Read the model definition and answer for the solid it produces. Units are mm, in the model's axes. Face numbers are marked on the shaded views. A direction names the side the tool comes from. Give positions to 0.01 mm unless a question says otherwise; leave off trailing zeros. Order: outer loops, then holes, each group sorted by start corner. A loop starts at its lowest first (then second) coordinate and runs counter-clockwise, first axis right, second up. Notation, with made-up numbers: (79, 0) - (96, 0) arc R16 cw to (96, 15) - close; hole circle Ø1 at (-25, 17). An arc over 180 degrees is marked (long way). Return JSON: item names as keys, results as strings.
Autodesk Inventor part; units mm, degrees
ref_plane "YZ Plane" through (0, 0, 0) normal (1, 0, 0) x (0, 1, 0)
ref_plane "XZ Plane" through (0, 0, 0) normal (0, 1, 0) x (-1, 0, 0)
ref_plane "XY Plane" through (0, 0, 0) normal (0, 0, 1) x (1, 0, 0)
sketch "草圖1" plane through (0, 0, 0) normal (0, 1, 0) x (-1, 0, 0)
  line L0 (0, 0) -> (44.45, 0)
  line L1 (44.45, 0) -> (44.45, -44.45)
  line L2 (44.45, -44.45) -> (0, -44.45)
  line L3 (0, -44.45) -> (0, 0)
  line L4 (3.725, -3.725) -> (40.725, -3.725)
  line L5 (40.725, -3.725) -> (40.725, -40.725)
  line L6 (40.725, -40.725) -> (3.725, -40.725)
  line L7 (3.725, -40.725) -> (3.725, -3.725)
  circle A0 centre (40.725, -3.725) radius 1.6
  circle A1 centre (40.725, -40.725) radius 1.6
  circle A2 centre (3.725, -3.725) radius 1.6
  circle A3 centre (3.725, -40.725) radius 1.6
  line L8 (11, -33.725) -> (0, -33.725)
  line L9 (0, -33.725) -> (0, -10.725)
  line L10 (0, -10.725) -> (11, -10.725)
  line L11 (11, -10.725) -> (11, -33.725)
  point P0 (0, -33.725)
  dimension "d0" = 44.45
  dimension "d1" = 44.45
  dimension "d2" = 37
  dimension "d3" = 37
  dimension "d4" = 3.725
  dimension "d5" = 3.725
  dimension "d6" = 3.2
  dimension "d7" = 3.2
  dimension "d8" = 3.2
  dimension "d9" = 3.2
  dimension "d14" = 23
  dimension "d15" = 11
  dimension "d16" = 10.725
extrude "擠出1" add sketch "草圖1" along normal blind 27 contours L10 L7 L8 L3 | L10 L11 L8 L7
extrude "擠出2" cut sketch "草圖1" along normal blind 27 contours A2 L4 L7 | L7 L4 A2 | A3 L6 L7 | L7 L6 A3 | A0 L5 L4 | L4 L5 A0 | A1 L5 L6 | L6 L5 A1
extrude "擠出3" add sketch "草圖1" along normal blind 1.6 contours L0 L1 L2 L3 L8 L7 A3 L6 A1 L5 A0 L4 A2 L10 | L7 A2 L4 A0 L5 A1 L6 A3 L8 L11 L10
properties part number "l298n"
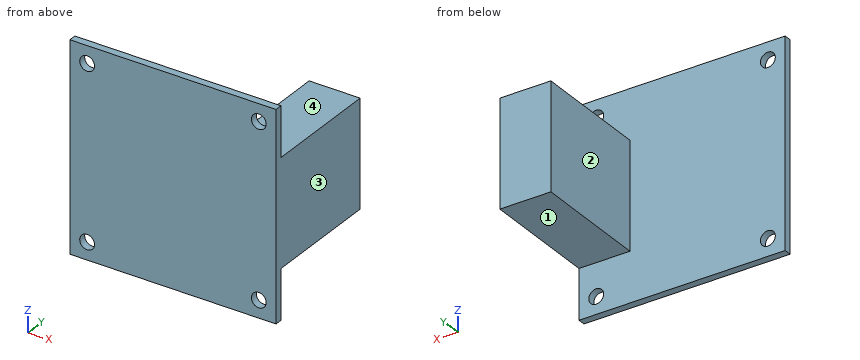
Q1. A cutting plane is placed at D-D (y = 10.75). Write down the section's boundary in (x, z) (3 decimals).
Values:
{"outline": "(-11, -33.725) - (0, -33.725) - (0, -10.725) - (-11, -10.725) - close"}
Q2. For the marked faces 1, 2, 3 and 4, determine the directions among +Z, -Z, +X, -X, +Y, -Y from which every point of the face is accessible in a straight line to the end or side of a thin tool.
Values:
{"face 1": "-Z, +X, -X, +Y", "face 2": "+Z, -Z, -X, +Y", "face 3": "+Z, -Z, +X, +Y, -Y", "face 4": "+Z, +X, -X, +Y"}
Q3. A cutting plane is placed at A-A (x = -4). Write down the section's boundary in (y, z) (3 decimals).
Values:
{"outline": "(0, -44.45) - (1.6, -44.45) - (1.6, -42.301) - (0, -42.301) - close; (0, -39.149) - (1.6, -39.149) - (1.6, -33.725) - (27, -33.725) - (27, -10.725) - (1.6, -10.725) - (1.6, -5.301) - (0, -5.301) - close; (0, -2.149) - (1.6, -2.149) - (1.6, 0) - (0, 0) - close"}
Q4. A cutting plane is placed at C-C (x = -38.5). Write down the section's boundary in (y, z), and give its area (3 significant figures).
Values:
{"outline": "(0, -44.45) - (1.6, -44.45) - (1.6, 0) - (0, 0) - close", "area": "71.1 mm²"}
Q5. Consider L1, parallel to Z at x = -40.5, y = 1.5; L2, parallel to Y at x = -33.5, z = -27; L3, parallel to Z at x = -5.5, y = 26 (3 decimals). Determine where each line is inside the solid, lowest interval first.
Values:
{"L1": "z = -44.45 to -42.31, -39.14 to -5.31, -2.14 to 0", "L2": "y = 0 to 1.6", "L3": "z = -33.725 to -10.725"}
Q6. Given pin 1 (1 mm diameter, centred on x = -29.5, z = -21.5, fed in from +Y); pin 2 (1.5 mm diameter, centred on x = -11.5, y = 9, fed in from -Z) (3 decimals); pin 3 (2 mm diameter, centred on y = 15.5, z = -12, fed in from -X), each flat-ended and moving along its own axis, determine where each tip first touches the part or whether it passes through.
Values:
{"pin 1": "stops at y = 1.6", "pin 2": "stops at z = -33.725", "pin 3": "stops at x = -11"}
Q7. A cutting plane is placed at B-B (z = -30.5). Write down the section's boundary in (x, y), and give its area (3 significant figures).
Values:
{"outline": "(-44.45, 0) - (0, 0) - (0, 27) - (-11, 27) - (-11, 1.6) - (-44.45, 1.6) - close", "area": "351 mm²"}
